Source: CAD feature listing. Evaluate the final solid. Frame: model axes, mm. A direction names the side the tool comes from. Give positions to 0.01 mm unless a question says otherwise; leave off trailing zeros. Write each loop counter-clockwise with the first axis right and the second up, starting at its lowest first coordinate (ties: lowest second). Pieces come first, ordered by that corner, then holes. Notation, with made-up numbers: (79, 68) -> (129, 68) arc R16 ccw to (129, 95) -> close; hole circle Ø9 at (51.5, 62). An arc over 180 degrees is marked (long way). Use a Markdown table: item, result. Add a question column.
```python
from build123d import *

# Parameters (mm, degrees)
SKETCH1_W               = 279.4
SKETCH1_H               = 279.4
BOSS_EXTRUDE1_DEPTH     = 12.7
SKETCH2_W               = 25.4
SKETCH2_H               = 12.7
BOSS_EXTRUDE2_DEPTH     = 12.7
LPATTERN1_COUNT         = 6
LPATTERN1_PITCH         = 50.8
MIRROR1_COPY_1_SKETCH_W = 25.4
MIRROR1_COPY_1_SKETCH_H = 12.7
MIRROR1_COPY_1_DEPTH    = 12.7
MIRROR1_COPY_2_SKETCH_W = 25.4
MIRROR1_COPY_2_SKETCH_H = 12.7
MIRROR1_COPY_2_DEPTH    = 12.7
MIRROR1_COPY_3_SKETCH_W = 25.4
MIRROR1_COPY_3_SKETCH_H = 12.7
MIRROR1_COPY_3_DEPTH    = 12.7
MIRROR1_COPY_4_SKETCH_W = 25.4
MIRROR1_COPY_4_SKETCH_H = 12.7
MIRROR1_COPY_4_DEPTH    = 12.7
MIRROR1_COPY_5_SKETCH_W = 25.4
MIRROR1_COPY_5_SKETCH_H = 12.7
MIRROR1_COPY_5_DEPTH    = 12.7
SKETCH3_W               = 25.4
SKETCH3_H               = 12.7
BOSS_EXTRUDE3_DEPTH     = 12.7
LPATTERN2_COUNT         = 6
LPATTERN2_PITCH         = 50.8
SKETCH5_W               = 17.00363529
SKETCH5_H               = 12.7
BOSS_EXTRUDE4_DEPTH     = 12.7
SKETCH6_R               = 44.45
CUT_EXTRUDE1_DEPTH      = 13.7
SKETCH7_R               = 5.715
CUT_EXTRUDE2_DEPTH      = 13.7
SKETCH8_R               = 2.1
CUT_EXTRUDE3_DEPTH      = 13.7


with BuildPart() as part:
    # Sketch1 → Boss-Extrude1 (new body)
    with BuildSketch(Plane(origin=(0, 0, 0), x_dir=(1, 0, 0), z_dir=(0, 1, 0))):
        Rectangle(SKETCH1_W, SKETCH1_H)
    extrude(amount=BOSS_EXTRUDE1_DEPTH)

    # Sketch2 → Boss-Extrude2 (add)
    with BuildSketch(Plane(origin=(139.7, 0, 0), x_dir=(0, 0, -1), z_dir=(1, 0, 0))):
        with Locations((-127, 6.35)):
            Rectangle(SKETCH2_W, SKETCH2_H)
    boss_extrude2 = extrude(amount=BOSS_EXTRUDE2_DEPTH)

    # LPattern1: Boss-Extrude2 ×6
    with Locations(*[(0, 0, -i * LPATTERN1_PITCH) for i in range(1, LPATTERN1_COUNT)]):
        add(boss_extrude2)

    # Mirror1: Boss-Extrude2 across plane
    add(boss_extrude2.mirror(Plane(origin=(0, 0, 0), x_dir=(0, 0, 1), z_dir=(1, 0, 0))))

    # Mirror1 copy 1 sketch → Mirror1 copy 1 (add)
    with BuildSketch(Plane(origin=(-139.7, 0, -50.8), x_dir=(0, 0, -1), z_dir=(-1, 0, 0))):
        with Locations((-127, -6.35)):
            Rectangle(MIRROR1_COPY_1_SKETCH_W, MIRROR1_COPY_1_SKETCH_H)
    extrude(amount=MIRROR1_COPY_1_DEPTH)

    # Mirror1 copy 2 sketch → Mirror1 copy 2 (add)
    with BuildSketch(Plane(origin=(-139.7, 0, -101.6), x_dir=(0, 0, -1), z_dir=(-1, 0, 0))):
        with Locations((-127, -6.35)):
            Rectangle(MIRROR1_COPY_2_SKETCH_W, MIRROR1_COPY_2_SKETCH_H)
    extrude(amount=MIRROR1_COPY_2_DEPTH)

    # Mirror1 copy 3 sketch → Mirror1 copy 3 (add)
    with BuildSketch(Plane(origin=(-139.7, 0, -152.4), x_dir=(0, 0, -1), z_dir=(-1, 0, 0))):
        with Locations((-127, -6.35)):
            Rectangle(MIRROR1_COPY_3_SKETCH_W, MIRROR1_COPY_3_SKETCH_H)
    extrude(amount=MIRROR1_COPY_3_DEPTH)

    # Mirror1 copy 4 sketch → Mirror1 copy 4 (add)
    with BuildSketch(Plane(origin=(-139.7, 0, -203.2), x_dir=(0, 0, -1), z_dir=(-1, 0, 0))):
        with Locations((-127, -6.35)):
            Rectangle(MIRROR1_COPY_4_SKETCH_W, MIRROR1_COPY_4_SKETCH_H)
    extrude(amount=MIRROR1_COPY_4_DEPTH)

    # Mirror1 copy 5 sketch → Mirror1 copy 5 (add)
    with BuildSketch(Plane(origin=(-139.7, 0, -254), x_dir=(0, 0, -1), z_dir=(-1, 0, 0))):
        with Locations((-127, -6.35)):
            Rectangle(MIRROR1_COPY_5_SKETCH_W, MIRROR1_COPY_5_SKETCH_H)
    extrude(amount=MIRROR1_COPY_5_DEPTH)

    # Sketch3 → Boss-Extrude3 (add)
    with BuildSketch(Plane(origin=(0, 0, -139.7), x_dir=(-1, 0, 0), z_dir=(0, 0, -1))):
        with Locations((-130.175, 6.35)):
            Rectangle(SKETCH3_W, SKETCH3_H)
    boss_extrude3 = extrude(amount=BOSS_EXTRUDE3_DEPTH)

    # LPattern2: Boss-Extrude3 ×6
    with Locations(*[(-i * LPATTERN2_PITCH, 0, 0) for i in range(1, LPATTERN2_COUNT)]):
        add(boss_extrude3)

    # Sketch5 → Boss-Extrude4 (add)
    with BuildSketch(Plane(origin=(0, 0, -139.7), x_dir=(-1, 0, 0), z_dir=(0, 0, -1))):
        with Locations((-143.898182355, 6.35)):
            Rectangle(SKETCH5_W, SKETCH5_H)
    boss_extrude4 = extrude(amount=BOSS_EXTRUDE4_DEPTH)

    # Mirror2: Boss-Extrude4 across plane
    add(boss_extrude4.mirror(Plane(origin=(0, 0, 0), x_dir=(0, 0, 1), z_dir=(1, 0, 0))))

    # Sketch6 → Cut-Extrude1 (cut, through all)
    with BuildSketch(Plane(origin=(0, 12.7, 0), x_dir=(1, 0, 0), z_dir=(0, 1, 0))):
        with Locations((38.1, 11.176)):
            Circle(SKETCH6_R)
    extrude(amount=-CUT_EXTRUDE1_DEPTH, mode=Mode.SUBTRACT)

    # Sketch7 → Cut-Extrude2 (cut, through all)
    with BuildSketch(Plane(origin=(0, 12.7, 0), x_dir=(1, 0, 0), z_dir=(0, 1, 0))):
        with Locations((-101.6, 65.278)):
            Circle(SKETCH7_R)
        with Locations((-101.6, 27.686)):
            Circle(SKETCH7_R)
    extrude(amount=-CUT_EXTRUDE2_DEPTH, mode=Mode.SUBTRACT)

    # Sketch8 → Cut-Extrude3 (cut, through all)
    with BuildSketch(Plane(origin=(0, 12.7, 0), x_dir=(1, 0, 0), z_dir=(0, 1, 0))):
        with Locations((-100.9, -81.986081859)):
            Circle(SKETCH8_R)
        with Locations((-100.9, -16.378881859)):
            Circle(SKETCH8_R)
    extrude(amount=-CUT_EXTRUDE3_DEPTH, mode=Mode.SUBTRACT)


solid = part.part
```
(1) Material intervals for L1, parallel to Z at x = -100.9, y = 8; L2, parallel to Z at x = -101.6, y = 6.5; L3, parallel to Z at x = -96.5, y = 9.75 (3 decimals), sorted ascending.
(2) Cut plane A-A on x = 53. Return the cut outline in (y, z), then the cut area to 3 significant figures.
(3) Cut plane C-C on z = -95. Return the cut outline in (x, y).
(4) Cut plane D-D on y = 8. Count the separate pieces of the cut face and the enclosed holes in it, then the cut area to 3 significant figures.
(5) Access query for faces 5 (the flat face through (-98, 6, -139.7)), 6 (the flat face through (146, 6, 12.7)), 7 (the flat face through (-139.7, 6, -101)), 8 (the flat face through (-152.4, 6, 76)). Directions: +Z, -Z, +X, -X, +Y, -Y. A direction counts if a zero-diameter tool reaches every point of the face in a straight line with its end or side. Return the directions, or none.
(6) Mould query, pull axis Z, two halves, no side actions, for faces 1 (the flat face through (-139.7, 6, -51)), 2 (the flat face through (-2, 0, 28)), 3 (the flat face through (-139.7, 6, 102)), 4 (the flat face through (29, 6, -152.4)). Classes: +Z half, -Z half, draft (parallel to the pull), parting line (faces both ways), or undercut.
(7) Cut plane B-B on z = -0.5. Return the cut outline in (x, y), then the cut area to 3 significant figures.
Output:
| question | item | result |
|---|---|---|
| 1 | L1 | -139.7 to -70.95, -59.61 to -33.36, -22.01 to 14.28, 18.48 to 79.89, 84.09 to 139.7 |
| 1 | L2 | -139.7 to -70.99, -59.56 to -33.4, -21.97 to 14.4, 18.36 to 80.01, 83.97 to 139.7 |
| 1 | L3 | -139.7 to -67.857, -62.699 to -30.265, -25.107 to 139.7 |
| 2 | outline | (0, -139.7) -> (12.7, -139.7) -> (12.7, -53.05) -> (0, -53.05) -> close; (0, 30.7) -> (12.7, 30.7) -> (12.7, 139.7) -> (0, 139.7) -> close |
| 2 | area | 2,480 mm^2 |
| 3 | outline | (-139.7, 0) -> (139.7, 0) -> (139.7, 12.7) -> (-139.7, 12.7) -> close |
| 4 | separate pieces | 1 |
| 4 | enclosed holes | 5 |
| 4 | area | 77,800 mm^2 |
| 5 | face 5 | -Z, +Y, -Y |
| 5 | face 6 | +X, +Y, -Y |
| 5 | face 7 | -X, +Y, -Y |
| 5 | face 8 | +Z, -Z, -X, +Y, -Y |
| 6 | face 1 | undercut |
| 6 | face 2 | draft |
| 6 | face 3 | undercut |
| 6 | face 4 | -Z half |
| 7 | outline | (-139.7, 0) -> (-5.05, 0) -> (-5.05, 12.7) -> (-139.7, 12.7) -> close; (81.25, 0) -> (139.7, 0) -> (139.7, 12.7) -> (81.25, 12.7) -> close |
| 7 | area | 2,450 mm^2 |
